Part model, mm, in its own coordinate system. A direction names the side the tool comes from. Coordinates: 2 decimals unless noted, no trailing zeros. Order: outer loops, then holes, each group sorted by start corner. A loop starts at its lowest first (then second) coordinate and runs counter-clockwise, first axis right, second up. Notation, with made-up numbers: (38, 22) - (46, 22) arc R33 cw to (46, 57) - close; hole circle Ø6 at (35, -6). An arc over 180 degrees is marked (long way). Use a Markdown table: item, result. Add a question column.
1) Two-plate mould, pull along Y, no slides. Class faces 6 (the face through (89, 60, 30)), 7 (the face through (5, 30, 36)), 8 (the face through (0, 30, 36)): +Y half, -Y half, draft (parallel to the pull), parting line (faces both ways), or undercut.
2) Saw through at B-B on z = 14.5. List the corners of the cut face in (x, y).
3) Saw through at A-A on x = 70. List the corners of the cut face in (y, z), then the cut area to 3 significant figures.
4) Tool access for faces 1 (the face through (177.46, 32.11, 38.66)), 2 (the face through (73, 3, 49)), 3 (the face through (2, 40, 15)), 4 (the face through (90, 3, 0)), 5 (the face through (89, 55, 27)): list every direction of +Z, -Z, +X, -X, +Y, -Y with a clear straight run to the whole face (end or side of a thin tool).
5) Wall check: L1, parallel to Z at x = 153.5, y = 1.65; L2, parallel to X at y = 1.6, z = 30.7; L3, parallel to Z at x = 90, y = 2. Give the ranges that are in metal, low to high. Write a range as [from, to].
6) Saw through at C-C on x = 47.5. List the corners of the cut face in (y, z), then the cut area to 3 significant figures.
7) Drop flat-ended pins along their axis: P1, Ø1.5, axis at x = 66.5, y = 42.5, coming from the -Z side; P2, Ø1.8, axis at x = 153.5, z = 19.3, coming from the -Y side; P3, Ø5.5, axis at x = 178, y = 26, coming from the -Z side. Give the stop position or say it passes through.
8) Saw through at D-D on y = 30. List the corners of the cut face in (x, z).
```python
from build123d import *

# Parameters (mm, degrees)
CYLINDER010_R     = 5
CYLINDER010_DEPTH = 5
CYLINDER009_R     = 5
CYLINDER009_DEPTH = 5
CYLINDER008_R     = 5
CYLINDER008_DEPTH = 5
CYLINDER005_R     = 1
CYLINDER005_DEPTH = 13
CYLINDER006_R     = 1
CYLINDER006_DEPTH = 13
CYLINDER007_R     = 1
CYLINDER007_DEPTH = 13
CYLINDER004_R     = 1
CYLINDER004_DEPTH = 13
CYLINDER_R        = 2.5
CYLINDER_DEPTH    = 180
BOX003_W          = 170
BOX003_H          = 15
BOX003_DEPTH      = 5
BOX002_W          = 180
BOX002_H          = 20
BOX002_DEPTH      = 30
BOX_W             = 170
BOX_H             = 50
BOX_DEPTH         = 55
BOX001_W          = 180
BOX001_H          = 60
BOX001_DEPTH      = 60


with BuildPart() as led3:
    # Cylinder010 → Cylinder010 (new body)
    with BuildSketch(Plane(origin=(110, 5, 45), x_dir=(1, 0, 0), z_dir=(0, -1, 0))):
        Circle(CYLINDER010_R)
    extrude(amount=CYLINDER010_DEPTH)


with BuildPart() as led2:
    # Cylinder009 → Cylinder009 (new body)
    with BuildSketch(Plane(origin=(70, 5, 45), x_dir=(1, 0, 0), z_dir=(0, -1, 0))):
        Circle(CYLINDER009_R)
    extrude(amount=CYLINDER009_DEPTH)


with BuildPart() as leds:
    # Cylinder008 → Cylinder008 (new body)
    with BuildSketch(Plane(origin=(90, 5, 45), x_dir=(1, 0, 0), z_dir=(0, -1, 0))):
        Circle(CYLINDER008_R)
    extrude(amount=CYLINDER008_DEPTH)

    # Fusion002: union LED3, LED2
    add(led3.part)
    add(led2.part)


with BuildPart() as topleft:
    # Cylinder005 → Cylinder005 (new body)
    with BuildSketch(Plane(origin=(106.5, 14, 30.7), x_dir=(1, 0, 0), z_dir=(0, -1, 0))):
        Circle(CYLINDER005_R)
    extrude(amount=CYLINDER005_DEPTH)


with BuildPart() as bottomright:
    # Cylinder006 → Cylinder006 (new body)
    with BuildSketch(Plane(origin=(153.5, 14, 19.3), x_dir=(1, 0, 0), z_dir=(0, -1, 0))):
        Circle(CYLINDER006_R)
    extrude(amount=CYLINDER006_DEPTH)


with BuildPart() as bottomleft:
    # Cylinder007 → Cylinder007 (new body)
    with BuildSketch(Plane(origin=(153.5, 14, 30.7), x_dir=(1, 0, 0), z_dir=(0, -1, 0))):
        Circle(CYLINDER007_R)
    extrude(amount=CYLINDER007_DEPTH)


with BuildPart() as fusion001:
    # Cylinder004 → Cylinder004 (new body)
    with BuildSketch(Plane(origin=(106.5, 14, 19.3), x_dir=(1, 0, 0), z_dir=(0, -1, 0))):
        Circle(CYLINDER004_R)
    extrude(amount=CYLINDER004_DEPTH)

    # Fusion001: union TopLeft, BottomRight, BottomLeft
    add(topleft.part)
    add(bottomright.part)
    add(bottomleft.part)


with BuildPart() as fusion001_1:
    # Fusion001 placement: moved
    add(fusion001.part.moved(Location((0, -1, 0))))


with BuildPart() as cylinder:
    # Cylinder → Cylinder (new body)
    with BuildSketch(Plane(origin=(0, 30, 40), x_dir=(0, 0, -1), z_dir=(1, 0, 0))):
        Circle(CYLINDER_R)
    extrude(amount=CYLINDER_DEPTH)


with BuildPart() as cube003:
    # Box003 → Box003 (new body)
    with BuildSketch(Plane(origin=(5, 22.5, 55), x_dir=(1, 0, 0), z_dir=(0, 0, 1))):
        with Locations((85, 7.5)):
            Rectangle(BOX003_W, BOX003_H)
    extrude(amount=BOX003_DEPTH)


with BuildPart() as cube002:
    # Box002 → Box002 (new body)
    with BuildSketch(Plane(origin=(0, 20, 0), x_dir=(1, 0, 0), z_dir=(0, 0, 1))):
        with Locations((90, 10)):
            Rectangle(BOX002_W, BOX002_H)
    extrude(amount=BOX002_DEPTH)


with BuildPart() as cube:
    # Box → Box (new body)
    with BuildSketch(Plane(origin=(5, 5, 0), x_dir=(1, 0, 0), z_dir=(0, 0, 1))):
        with Locations((85, 25)):
            Rectangle(BOX_W, BOX_H)
    extrude(amount=BOX_DEPTH)


with BuildPart() as cut007:
    # Box001 → Box001 (new body)
    with BuildSketch(Plane.XY):
        with Locations((90, 30)):
            Rectangle(BOX001_W, BOX001_H)
    extrude(amount=BOX001_DEPTH)

    # Cut: cut Cube
    add(cube.part, mode=Mode.SUBTRACT)

    # Cut001: cut Cube002
    add(cube002.part, mode=Mode.SUBTRACT)

    # Cut002: cut Cube003
    add(cube003.part, mode=Mode.SUBTRACT)

    # Cut003: cut Cylinder
    add(cylinder.part, mode=Mode.SUBTRACT)

    # Cut006: cut Fusion001
    add(fusion001_1.part, mode=Mode.SUBTRACT)

    # Cut007: cut LEDs
    add(leds.part, mode=Mode.SUBTRACT)


solid = cut007.part
```
Results are:
| question | item | result |
|---|---|---|
| 1 | face 6 | +Y half |
| 1 | face 7 | undercut |
| 1 | face 8 | draft |
| 2 | outline | (0, 0) - (180, 0) - (180, 20) - (175, 20) - (175, 5) - (5, 5) - (5, 20) - (0, 20) - close; (0, 40) - (5, 40) - (5, 55) - (175, 55) - (175, 40) - (180, 40) - (180, 60) - (0, 60) - close |
| 3 | outline | (0, 0) - (5, 0) - (5, 40) - (0, 40) - close; (0, 50) - (5, 50) - (5, 55) - (22.5, 55) - (22.5, 60) - (0, 60) - close; (37.5, 55) - (55, 55) - (55, 0) - (60, 0) - (60, 60) - (37.5, 60) - close |
| 3 | area | 725 mm2 |
| 4 | face 1 | +X, -X |
| 4 | face 2 | -Y |
| 4 | face 3 | -Z, +X, -X |
| 4 | face 4 | -Z, +X, -X, +Y, -Y |
| 4 | face 5 | -Z |
| 5 | L1 | [0, 18.3], [20.3, 29.7], [31.7, 60] |
| 5 | L2 | [0, 105.5], [107.5, 152.5], [154.5, 180] |
| 5 | L3 | [0, 40], [50, 60] |
| 6 | outline | (0, 0) - (5, 0) - (5, 55) - (22.5, 55) - (22.5, 60) - (0, 60) - close; (37.5, 55) - (55, 55) - (55, 0) - (60, 0) - (60, 60) - (37.5, 60) - close |
| 6 | area | 775 mm2 |
| 7 | P1 | z = 55 |
| 7 | P2 | y = 55 |
| 7 | P3 | z = 30 |
| 8 | outline | (0, 30) - (5, 30) - (5, 37.5) - (0, 37.5) - close; (0, 42.5) - (5, 42.5) - (5, 60) - (0, 60) - close; (175, 30) - (180, 30) - (180, 37.5) - (175, 37.5) - close; (175, 42.5) - (180, 42.5) - (180, 60) - (175, 60) - close |
